Input: part model. Units: mm. Frame: model coordinates. A direction names the side the tool comes from. Give positions to 0.01 mm unless a question says otherwise; leave off trailing zeros. Loops run counter-clockwise (first coordinate to the right, second up) from the corner with the lowest first, then second, coordinate; pieces in that order, holes last. Notation, with made-up numbers: M 47.5,70 L 91.5,70 A21 cw 91.5,90 Z; hole C 81,-12 d11. An arc over 180 degrees is marked long. One line per item, written item: value. Start each with the question number.
(1) Pin query (flat end, axial travel): P1, Ø10, axis at y = 32, z = 9, coming from the +X side; P2, Ø4, axis at x = 15.5, z = 2.5, coming from the +Y side; P3, Ø5, axis at x = 25, z = -3.5, coming from the -Y side; P4, Ø11, axis at x = -3, y = 27, coming from the -Z side. Return the tip coordinate at first contact, or that it passes through.
(2) Section C-C on z = 13.5. Output: boundary loops of the cut face in (x, y).
(3) Section B-B on z = -3.5. Output: boundary loops of the cut face in (x, y).
(4) Section D-D on x = -5. Output: boundary loops of the cut face in (y, z).
(5) Pull-direction query (X, two-part tool) for faces 3 (the cylindrical face through (26.265, 1.972, -4.306)), 4 (the flat face through (0, 20, 9)), 5 (the flat face through (15, 2, -1)); classes: released by +X, released by -X, zero draft, split by the parting line, or undercut.
(6) Access query for faces 1 (the flat face through (-6.451, 29.154, 9.86)), 2 (the flat face through (10, 4, -4)). Directions: +Z, -Z, +X, -X, +Y, -Y. A direction counts if a zero-diameter tool reaches every point of the face in a straight line with its end or side. Return the directions, or none.
(7) Ray query, line 1 along X through (y, z) = (2.5, -3.5); line 2 along Z through (x, y) = (-2.5, 11.5); line 3 along X through (y, z) = (17, 11). Return the intervals inside material, ascending. Write a range as from..to.
(8) Section A-A on x = 25. Output: boundary loops of the cut face in (y, z), plus the area to 3 significant figures.
```python
from build123d import *

# Parameters (mm, degrees)
BOSS_EXTRUDE1_DEPTH = 20
SKETCH2_R           = 1.5
BOSS_EXTRUDE2_DEPTH = 4


with BuildPart() as part:
    # Sketch1 → Boss-Extrude1 (new body)
    with BuildSketch(Plane.XY):
        Polygon((0, 0), (0, 40), (-3, 40), (-10, 18), (-10, 0), align=None)
    extrude(amount=BOSS_EXTRUDE1_DEPTH)

    # Sketch2 → Boss-Extrude2 (add)
    with BuildSketch(Plane.XZ):
        Polygon((-10, 0), (-10, -6), (30, -6), (30, -1), (0, -1), (0, 0), align=None)
        with Locations(Location((25, -3.5, 0), (0, 0, 270))):
            Circle(SKETCH2_R, mode=Mode.SUBTRACT)
        with Locations(Location((-5, -3.5, 0), (0, 0, 270))):
            Circle(SKETCH2_R, mode=Mode.SUBTRACT)
    extrude(amount=-BOSS_EXTRUDE2_DEPTH)


solid = part.part
```
Output values:
1. P1: stops at x = 0
1. P2: passes through
1. P3: stops at y = 0
1. P4: stops at z = 0
2. outline: M -10,0 L 0,0 L 0,40 L -3,40 L -10,18 Z
3. outline: M -10,0 L -6.5,0 L -6.5,4 L -10,4 Z; M -3.5,0 L 23.5,0 L 23.5,4 L -3.5,4 Z; M 26.5,0 L 30,0 L 30,4 L 26.5,4 Z
4. outline: M 0,-6 L 4,-6 L 4,-5 L 0,-5 Z; M 0,-2 L 4,-2 L 4,0 L 33.71,0 L 33.71,20 L 0,20 Z
5. face 3: undercut
5. face 4: released by +X
5. face 5: zero draft
6. face 1: +Z, -Z, -X, +Y
6. face 2: -Z, +X, -X, +Y
7. line 1: x = -10..-6.5, -3.5..23.5, 26.5..30
7. line 2: z = 0..20
7. line 3: x = -10..0
8. outline: M 0,-6 L 4,-6 L 4,-5 L 0,-5 Z; M 0,-2 L 4,-2 L 4,-1 L 0,-1 Z
8. area: 8.00 mm²
